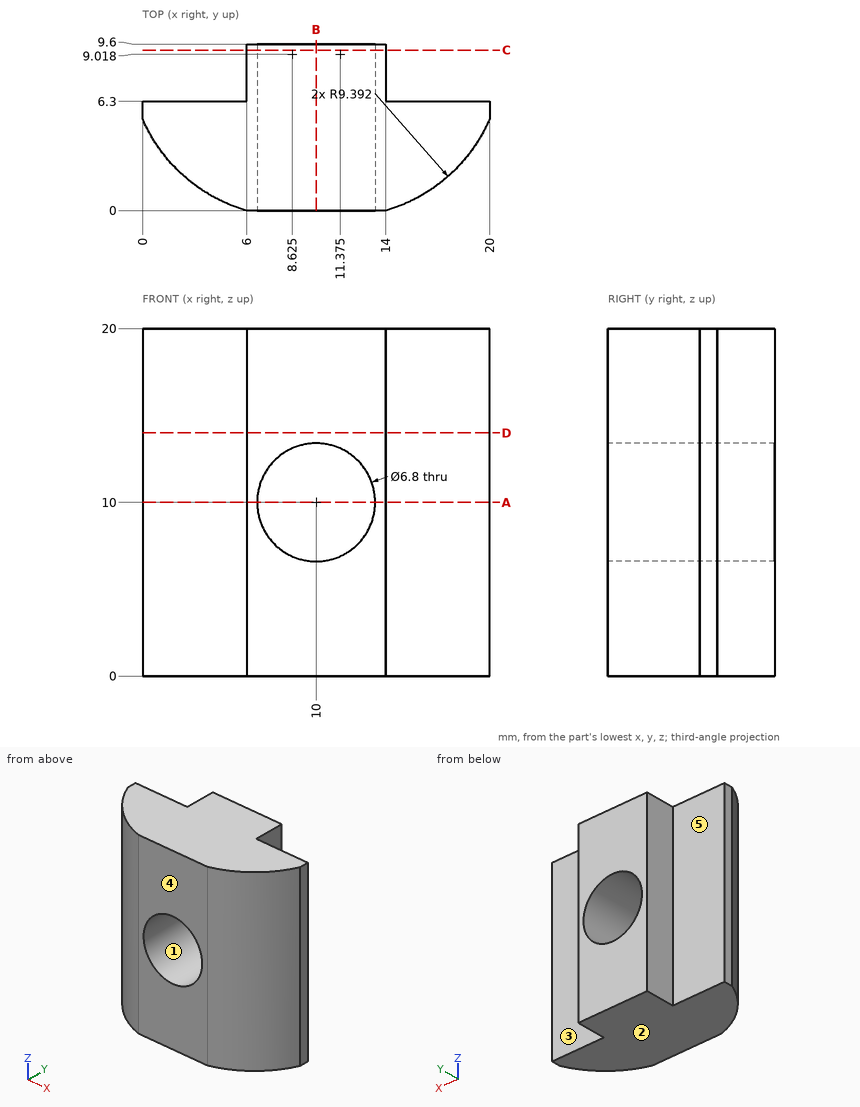
Geometry check sheet. Reference: drawing and pictorial views, mm from the part's lowest x, y, z. A direction names the side the tool comes from. Coordinates: 2 decimals unless noted, no trailing zeros. Order: outer loops, then holes, each group sorted by start corner. A loop starts at its lowest first (then second) coordinate and runs counter-clockwise, first axis right, second up.
Item 1: Section check C-C (y = 9.25). Enter the section's corners in (x, z), plus the area to 3 significant figures.
Item 2: Section check D-D (z = 14). Enter the section's corners in (x, y) (1 decimal), plus the area to 3 significant figures.
Item 3: Tool access check on the marked faces 4 and 5. Record the directions out of +Z, -Z, +X, -X, +Y, -Y that give a thin tool (end or side, any length) a straight path to the whole face; none if there is none.
Item 4: Section check B-B (x = 10). Enter the section's corners in (y, z), plus the area to 3 significant figures.
Item 5: Depth check by flat-ended pin: pin 1 (3 mm diameter, centred on x = 2, z = 8.5, fed in from +Y); pin 2 (1 mm diameter, centred on y = 8, z = 8.5, fed in from -X); pin 3 (2.5 mm diameter, centred on y = 8.5, z = 8, fed in from +X). Enter the tip coordinate at first touch or a pass-through.
Item 6: Section check A-A (z = 10). Enter the section's corners in (x, y) (1 decimal).
Item 7: Scan lines: line 1 along X through (y, z) = (7.25, 10); line 2 along X through (y, z) = (4.5, 10); line 3 along X through (y, z) = (6.5, 13.75). Record each from-to range of solid material in increasing order.
Item 8: Mould release check, pull along Z, two halves, no side actions. Record for the marked faces 1, 2 and 3: released by +Z, released by -Z, zero draft, split by the parting line, or undercut.
Check sheet entries:
1. outline: (6, 0) - (14, 0) - (14, 20) - (6, 20) - close; hole circle Ø6.8 at (10, 10)
1. area: 124 mm2
2. outline: (0, 5.3) arc R9.4 ccw to (6, 0) - (14, 0) arc R9.4 ccw to (20, 5.3) - (20, 6.3) - (14, 6.3) - (14, 9.6) - (6, 9.6) - (6, 6.3) - (0, 6.3) - close
2. area: 130 mm2
3. face 4: +Z, -Z, +X, -X, -Y
3. face 5: +Z, -Z, -X, +Y
4. outline: (0, 0) - (9.6, 0) - (9.6, 6.6) - (0, 6.6) - close; (0, 13.4) - (9.6, 13.4) - (9.6, 20) - (0, 20) - close
4. area: 127 mm2
5. pin 1: stops at y = 6.3
5. pin 2: stops at x = 6
5. pin 3: stops at x = 14
6. outline: (0, 5.3) arc R9.4 ccw to (6, 0) - (6.6, 0) - (6.6, 9.6) - (6, 9.6) - (6, 6.3) - (0, 6.3) - close; (13.4, 0) - (14, 0) arc R9.4 ccw to (20, 5.3) - (20, 6.3) - (14, 6.3) - (14, 9.6) - (13.4, 9.6) - close
7. line 1: x = 6 to 6.6, 13.4 to 14
7. line 2: x = 0.39 to 6.6, 13.4 to 19.61
7. line 3: x = 6 to 14
8. face 1: undercut
8. face 2: released by -Z
8. face 3: zero draft
